```python
from build123d import *
from OCP.BRepFilletAPI import BRepFilletAPI_MakeChamfer

# Parameters (mm, degrees)
BOSS_EXTRUDE1_DEPTH = 4
CHAMFER1_SIZE       = 0.7
CHAMFER1_SIZE2      = 0.736453843


with BuildPart() as part:
    # Sketch1 → Boss-Extrude1 (new body)
    with BuildSketch(Plane.XY):
        Polygon((-10, 0), (0, 0), (0, 18.2), (-6.2, 18.5), (-6.2, 21.9), (0, 22.2), (0, 25.2), (-10, 25.2), align=None)
        Polygon((-6.2, -18.5), (0, -18.2), (0, 0), (-10, 0), (-10, -25.2), (0, -25.2), (0, -22.2), (-6.2, -21.9), align=None)
    extrude(amount=BOSS_EXTRUDE1_DEPTH)

    # Chamfer1: one chamfer whose edges measure the first distance from different faces: ONE call of the kernel's chamfer builder (chamfer() names one face for all edges)
    chamfer1_edges_1 = [part.edges().sort_by_distance(p)[0] for p in [
        (0, 22.2, 2),
    ]]
    chamfer1_side_1 = [part.faces().sort_by_distance(p)[0] for p in [
        (-3.1, 22.05, 2),
    ]]
    chamfer1_edges_2 = [part.edges().sort_by_distance(p)[0] for p in [
        (0, 18.2, 2),
    ]]
    chamfer1_side_2 = [part.faces().sort_by_distance(p)[0] for p in [
        (0, 0, 2),
    ]]
    chamfer1_edges_3 = [part.edges().sort_by_distance(p)[0] for p in [
        (0, -18.2, 2),
    ]]
    chamfer1_side_3 = [part.faces().sort_by_distance(p)[0] for p in [
        (-3.1, -18.35, 2),
    ]]
    chamfer1_edges_4 = [part.edges().sort_by_distance(p)[0] for p in [
        (0, -22.2, 2),
    ]]
    chamfer1_side_4 = [part.faces().sort_by_distance(p)[0] for p in [
        (0, -23.7, 2),
    ]]
    chamfer1 = BRepFilletAPI_MakeChamfer(part.part.solid().wrapped)
    for e in chamfer1_edges_1:
        chamfer1.Add(CHAMFER1_SIZE, CHAMFER1_SIZE2, e.wrapped, chamfer1_side_1[0].wrapped)  # the first distance lies on this face
    for e in chamfer1_edges_2:
        chamfer1.Add(CHAMFER1_SIZE, CHAMFER1_SIZE2, e.wrapped, chamfer1_side_2[0].wrapped)  # the first distance lies on this face
    for e in chamfer1_edges_3:
        chamfer1.Add(CHAMFER1_SIZE, CHAMFER1_SIZE2, e.wrapped, chamfer1_side_3[0].wrapped)  # the first distance lies on this face
    for e in chamfer1_edges_4:
        chamfer1.Add(CHAMFER1_SIZE, CHAMFER1_SIZE2, e.wrapped, chamfer1_side_4[0].wrapped)  # the first distance lies on this face
    add(Compound.cast(chamfer1.Shape()), mode=Mode.REPLACE)


solid = part.part
```
Part model, mm, in its own coordinate system. A direction names the side the tool comes from. Round coordinates to 2 decimals unless told otherwise and drop trailing zeros. Write each loop counter-clockwise with the first axis right and the second up, starting at its lowest first coordinate (ties: lowest second). Pieces come first, ordered by that corner, then holes. Notation, with made-up numbers: (11.25, 30.5) -> (60.25, 30.5) arc R28 ccw to (60.25, 58.5) -> close; hole circle Ø8 at (9.5, 68.25). An arc over 180 degrees is marked (long way). Return JSON: item names as keys, results as strings. Group by question number.
Q1. Mould opens along Y. For faces 1 (the flat face through (-6.2, 20, 2)), 2 (the flat face through (-5, 25.2, 2)), 3 (the flat face through (-10, 0, 2)), 4 (the flat face through (-5, -25.2, 2)) say: pulls with the +Y half, pulls with the -Y half, needs draft (parallel to the pull), parting line crosses it, or undercut.
Q2. Probe L1, parallel to Y at x = -6, z = 0.3; L2, parallel to Y at x = -2.5, z = 1.45; L3, parallel to X at y = 18, z = 2.25. List the from-to ranges inside material, lowest first. Write a range as [from, to].
Q3. Saw through at A-A on x = -4.5. Write the cut outline in (y, z), plus the area to 3 significant figures.
Q4. Which spindle directions (+Z, -Z, +X, -X, +Y, -Y) get a long thin tool onto all of the face, cutting with end or side? Do faces 5 (the flat face through (0, -24, 2)), 6 (the flat face through (-3.49, -18.37, 1.97)). Say none if no direction does.
Q5. Saw through at B-B on z = 2.65. Write the cut outline in (x, y).
Q6. Pin check, flat tip, straight feed: pin 1 (1.7 mm diameter, centred on y = 20, z = 1, fed in from +X). Stop position of the tip, or through.
Answer:
{
 "1": {"face 1": "undercut", "face 2": "pulls with the +Y half", "face 3": "needs draft", "face 4": "pulls with the -Y half"},
 "2": {"L1": "[-25.2, -21.91], [-18.49, 18.49], [21.91, 25.2]", "L2": "[-25.2, -22.08], [-18.32, 18.32], [22.08, 25.2]", "L3": "[-10, -0.5]"},
 "3": {"outline": "(-25.2, 0) -> (-21.98, 0) -> (-21.98, 4) -> (-25.2, 4) -> close; (-18.42, 0) -> (18.42, 0) -> (18.42, 4) -> (-18.42, 4) -> close; (21.98, 0) -> (25.2, 0) -> (25.2, 4) -> (21.98, 4) -> close", "area": "173 mm2"},
 "4": {"face 5": "+Z, -Z, +X, +Y, -Y", "face 6": "+Z, -Z, +X"},
 "5": {"outline": "(-10, -25.2) -> (0, -25.2) -> (0, -22.9) -> (-0.74, -22.16) -> (-6.2, -21.9) -> (-6.2, -18.5) -> (-0.7, -18.23) -> (0, -17.46) -> (0, 17.5) -> (-0.74, 18.24) -> (-6.2, 18.5) -> (-6.2, 21.9) -> (-0.7, 22.17) -> (0, 22.94) -> (0, 25.2) -> (-10, 25.2) -> close"},
 "6": {"pin 1": "x = -6.2"}
}
